Input: part model. Units: mm. Frame: model coordinates. Coordinates: 2 decimals unless noted, no trailing zeros. Loops run counter-clockwise (first coordinate to the right, second up) from the corner with the lowest first, then second, coordinate; pieces in that order, holes last. Notation, with made-up numbers: (52, 74.25) - (102, 74.25) arc R34 ccw to (102, 110.25) - close; hole circle Ø5 at (58, -10). An arc over 180 degrees is marked (long way). Use one line per item in the form item = value.
Autodesk Inventor part; units mm, degrees
ref_plane "YZ Plane" through (0, 0, 0) normal (1, 0, 0) x (0, 1, 0)
ref_plane "XZ Plane" through (0, 0, 0) normal (0, 1, 0) x (-1, 0, 0)
ref_plane "XY Plane" through (0, 0, 0) normal (0, 0, 1) x (1, 0, 0)
sketch "Sketch1" plane through (0, 0, 0) normal (0, 0, 1) x (1, 0, 0)
  line L0 (-5, -2.6054) -> (-5, 1.3946)
  line L1 (-5, -2.6054) -> (0, -2.6054)
  line L2 (0, -2.6054) -> (0, 7.3946)
  line L3 (0, 7.3946) -> (-2.8105, 7.3946)
  line L4 (-2.8105, 7.3946) -> (-5, 1.3946)
  point P0 (0, 0)
  dimension "d0" = 4
  dimension "d1" = 6
  dimension "d2" = 5
extrude "Extrusion1" add sketch "Sketch1" along normal blind 10
mirror "Mirror1" about plane through (0, 0, 0) normal (1, 0, 0) of "Extrusion1"
sketch "Sketch2" plane through (0, 0, 0) normal (1, 0, 0) x (0, 1, 0)
  line L0 (7.3946, 0) -> (7.3946, 10)
  line L1 (7.3946, 10) -> (1.3946, 10)
  line L2 (1.3946, 0) -> (1.3946, 10)
  arc A0 (7.3946, 8) -> (1.3946, 10) centre (1.3946, 0) ccw
  line L3 (7.3946, 0) -> (1.3946, 0)
  arc A1 (1.3946, 0) -> (7.3946, 2) centre (1.3946, 10) ccw
  point P0 (0, 0)
  dimension "d7" = 10
  dimension "d8" = 8
  dimension "d11" = 10
  dimension "d12" = 8
extrude "Extrusion3" cut sketch "Sketch2" along normal mid plane 10 contours L3 A1 L0 | A0 L1 L0
sketch "Sketch3" plane through (0, 0, 0) normal (1, 0, 0) x (0, 1, 0)
  line L0 (-2.6054, 0) -> (-2.6054, 10)
  line L1 (-2.6054, 10) -> (-2.6054, 14)
  line L2 (1.3946, 0) -> (1.3946, 10)
  arc A0 (-2.6054, 14) -> (1.3946, 10) centre (1.3946, 14) ccw
  line L3 (-2.6054, 0) -> (-2.6054, -4)
  line L4 (1.3946, 0) -> (-2.6054, 0)
  arc A1 (1.3946, 0) -> (-2.6054, -4) centre (3.9223, -6.5277) ccw
  arc A2 (7.3946, 8) -> (1.3946, 10) centre (1.3946, 0) ccw
  point P0 (0, 0)
  dimension "d15" = 4
  dimension "d17" = 7
  dimension "d18" = 4
extrude "Extrusion4" add sketch "Sketch3" along normal mid plane 10
equation "\"d2\" = rack_tooth_thickness"
equation "\"d3\" = rack_tooth_face_widh"
equation "\"d11\" = d7"
equation "\"d12\" = d8"
equation "\"d17\" = d16"
equation "\"d18\" = d15"
equation "\"rack_tooth_thickness\" = 5"
equation "\"rack_tooth_face_widh\" = 10"
equation "\"rack_tooth_addendum\" = 5"
equation "\"rack_tooth_dedendum\" = 5"
equation "\"hoop_width_large\" = 51"
equation "\"hoop_thickness_large\" = 4"
equation "\"hoop_thickness_small\" = 2"
equation "\"hoop_width_medium\" = 33.7"
equation "\"hoop_thickness_medium\" = 3.2"
equation "\"hoop_width_small\" = 25.4"
equation "\"secure_arm_angle\" = 35deg"
equation "\"secure_arm_radii\" = 9"
equation "\"hoop_bearing_length\" = 5deg"
equation "\"hoop_cable_pulley_diam\" = 22"
equation "\"hoop_cable_diam\" = 5"
equation "\"support_frame_squareBarThickness\" = 5"
equation "\"support_frame_squareBarFillet\" = 2"
equation "\"support_baseClamp_platformThickness\" = 15"
equation "\"support_baseClamp_platformWidthBuffer\" = 0"
equation "\"support_baseClamp_platformLengthBuffer\" = 35"
equation "\"support_frame_endHoleBuffer\" = 45"
equation "\"support_baseClamp_thickness\" = 8"
equation "\"support_baseClamp_sleeveSweepTerminationAngle\" = 55deg"
equation "\"support_baseClamp_sleeveHoleDiameter\" = 12"
equation "\"hoop_angle_z\" = 45deg"
equation "\"hoop_tabs_hole\" = 12"
equation "\"hoop_tabs_thickness\" = 6"
equation "\"wheelchair_deployed_width\" = 635"
equation "\"wheelchair_deployed_height\" = 914"
equation "\"wheelchair_deployed_length\" = 1067"
equation "\"sm_varx_member_tolerance\" = 0"
equation "\"sm_varx_pinPlate_holeDiameter\" = 5"
equation "\"sm_varx_pinPlate_thickness\" = 5"
equation "\"sm_varx_squareBarThickness\" = 2.5"
equation "\"hoop_bushing12_radialInterference\" = 0"
equation "\"hoop_bushing12_od\" = -2 * hoop_thickness_large + hoop_width_large + hoop_bushing12_radialInterference"
equation "\"hoop_bushing23_radialInterference\" = 0"
equation "\"hoop_bushing12_thickness\" = -hoop_width_medium + hoop_bushing12_od - 2 * hoop_bushing12_radialInterference"
equation "\"hoop_bushing23_od\" = -2 * hoop_thickness_medium + hoop_width_medium + hoop_bushing23_radialInterference"
equation "\"hoop_bushing23_thickness\" = -hoop_width_small + hoop_bushing23_od - 2 * hoop_bushing23_radialInterference"
equation "\"wheelchatir_pos_deploy_angle_0\" = 65deg"
equation "\"wheelchatir_pos_store_angle_0\" = 90deg"
equation "\"wheelchatir_pos_deploy_angle_1\" = 20deg"
equation "\"wheelchatir_pos_store_angle_1\" = 20deg"
properties part number "tooth" material "Steel, High Strength, Low Alloy"
Q1. Cut plane C-C, the plane y = 5.5. Return loops of the section in (x, z), then the cut area to 3 significant figures.
Check values:
outline = (-3.5, 0.88) - (3.5, 0.88) - (3.5, 9.12) - (-3.5, 9.12) - close
area = 57.7 mm²
Q2. Cut plane D-D, the plane y = 4. Return loops of the section in (x, z), then the cut area to 3 significant figures.
Check values:
outline = (-4.05, 0.35) - (4.05, 0.35) - (4.05, 9.65) - (-4.05, 9.65) - close
area = 75.4 mm²
Q3. Cut plane B-B, the plane x = 0.5. Return loops of the section in (y, z), then the cut area to 3 significant figures.
Check values:
outline = (-2.61, -4) arc R7 cw to (1.39, 0) arc R10 ccw to (7.39, 2) - (7.39, 8) arc R10 ccw to (1.39, 10) arc R4 cw to (-2.61, 14) - close
area = 102 mm²
Q4. Cut plane A-A, the plane z = 5.75. Return loops of the section in (x, y), then the cut area to 3 significant figures.
Check values:
outline = (-5, -2.61) - (5, -2.61) - (5, 1.39) - (2.81, 7.39) - (-2.81, 7.39) - (-5, 1.39) - close
area = 86.9 mm²
Q5. First-contact query: P1, Ø1.5, axis at x = -2, y = 3.5, coming from the +Z side; P2, Ø1.5, axis at x = -1, z = 9.5, coming from the +Y side; P3, Ø3, axis at y = 4, z = 10.5, coming from the -X side. Flat tips, straight axial feed; report the tip coordinate or a pass-through.
Check values:
P1 = 9.91
P2 = 6.24
P3 = -4.55
Q6. Ray query, line 1 along Z through (x, y) = (1.5, 3.5); line 2 along X through (y, z) = (6.5, 7.75); line 3 along Y through (x, z) = (-0.5, -2). Return the intervals inside material, ascending. Write a range as [from, to].
Check values:
line_1 = [0.22, 9.78]
line_2 = [-3.14, 3.14]
line_3 = [-2.61, -1.42]
